Model file for the job. Use its own axes, mm. A direction names the side the tool comes from. Round coordinates to 2 decimals unless told otherwise and drop trailing zeros. Order: outer loops, then holes, each group sorted by start corner. A loop starts at its lowest first (then second) coordinate and runs counter-clockwise, first axis right, second up. Notation, with made-up numbers: M -32.5,8.5 L -7.5,8.5 A14 ccw -7.5,17.5 Z; hole C -22,63.25 d5. An arc over 180 degrees is marked long. Return JSON: item names as keys, results as strings. Group by question number.
Item 1: Slice it at B-B on x = -3.25. Write the cut outline in (y, z).
Item 2: Slice it at C-C on z = 4.25. Write the cut outline in (x, y), then the cut area to 3 significant figures.
Item 3: Slice it at D-D on x = 4.5. Write the cut outline in (y, z), then the cut area to 3 significant figures.
Item 4: Probe line 1 along Y through (x, z) = (5.75, 0.9); line 2 along X through (y, z) = (1.75, 4.7); line 3 along Y through (x, z) = (-3.5, 1.35). List the from-to ranges inside material, lowest first.
Item 5: Pin check, flat tips, straight feed: pin 1 Ø1.2 at (y, z) = (3, 1.5) entering from -X; pin 2 Ø1.7 at (x, y) = (-1, 2) entering from -Z; pin 3 Ø1 at (x, z) = (0, 2) entering from -Y (3 decimals). Stop position of each tip, or through.
Item 6: Slice it at A-A on y = 2.5. Write the cut outline in (x, z), then the cut area to 3 significant figures.
Item 7: Which spindle directions (+Z, -Z, +X, -X, +Y, -Y) get a long thin tool onto all of the face, cutting with end or side? Do faces 1 (the face through (-0.25, 1.75, 5)), 2 (the face through (-2.7, 0.2, 2.3)), 3 (the face through (-3, 0.4, 4)), 4 (the face through (4, 6, 2)). Say none if no direction does.
from build123d import *

# Parameters (mm, degrees)
SM_BASE_FLANGE_1_DEPTH = 6
SKETCH_5_R             = 1
CUT_EXTRUDE_1_DEPTH    = 12.223190277
CUT_EXTRUDE_3_REACH    = 17.683
CUT_EXTRUDE_4_REACH    = 13.223


# Sheet-metal steps are written as plain solids
with BuildPart() as part:
    # Sketch 1 → 基体-法兰1 (new body)
    with BuildSketch(Plane.XY):
        with BuildLine():
            Line((-7, 0), (-1.1366, 0))
            ThreePointArc((-1.1366, 0), (-0.332902433, 0.332902433), (0, 1.1366))
            Line((0, 1.1366), (0, 5.2634))
            ThreePointArc((0, 5.2634), (0.215745145, 5.784254855), (0.7366, 6))
            Line((0.7366, 6), (6, 6))
            Line((6, 6), (6, 6.4))
            Line((6, 6.4), (0.7366, 6.4))
            ThreePointArc((0.7366, 6.4), (-0.067097567, 6.067097567), (-0.4, 5.2634))
            Line((-0.4, 5.2634), (-0.4, 1.1366))
            ThreePointArc((-0.4, 1.1366), (-0.615745145, 0.615745145), (-1.1366, 0.4))
            Line((-1.1366, 0.4), (-7, 0.4))
            Line((-7, 0.4), (-7, 0))
        make_face()
    extrude(amount=SM_BASE_FLANGE_1_DEPTH)

    # 草图5 → 切除-拉伸1 (cut, through all)
    with BuildSketch(Plane(origin=(0, 6.4, 0), x_dir=(1, 0, 0), z_dir=(0, 1, 0))):
        with Locations(Location((2.913465792, -3, 0), (0, 0, 270))):
            Circle(SKETCH_5_R)
    extrude(amount=-CUT_EXTRUDE_1_DEPTH, mode=Mode.SUBTRACT)

    # 草图6 → 切除-拉伸3 (cut, up to next)
    with BuildSketch(Plane.ZY.offset(7), mode=Mode.PRIVATE) as cut_extrude_3_sk1:
        with BuildLine():
            Line((2.3, -3.316111615), (2.3, 3.5366))
            ThreePointArc((2.3, 3.5366), (2.475735931, 3.960864069), (2.9, 4.1366))
            Line((2.9, 4.1366), (3, 4.1366))
            Line((3, 4.1366), (3.1, 4.1366))
            ThreePointArc((3.1, 4.1366), (3.524264069, 3.960864069), (3.7, 3.5366))
            Line((3.7, 3.5366), (3.7, -3.316111615))
            Line((3.7, -3.316111615), (2.3, -3.316111615))
        make_face()
    cut_extrude_3_tool1 = extrude(cut_extrude_3_sk1.sketch, amount=-CUT_EXTRUDE_3_REACH, mode=Mode.PRIVATE) & part.part
    # 草图6 → 切除-拉伸3 (cut, up to next)
    with BuildSketch(Plane.ZY.offset(7), mode=Mode.PRIVATE) as cut_extrude_3_sk2:
        Polygon((1, -3.316111615), (1, 4.1366), (0, 4.629449722), (0, -3.316111615), align=None)
    cut_extrude_3_tool2 = extrude(cut_extrude_3_sk2.sketch, amount=-CUT_EXTRUDE_3_REACH, mode=Mode.PRIVATE) & part.part
    # 草图6 → 切除-拉伸3 (cut, up to next)
    with BuildSketch(Plane.ZY.offset(7), mode=Mode.PRIVATE) as cut_extrude_3_sk3:
        Polygon((5, 4.1366), (6, 4.629449722), (6, -3.316111615), (5, -3.316111615), align=None)
    cut_extrude_3_tool3 = extrude(cut_extrude_3_sk3.sketch, amount=-CUT_EXTRUDE_3_REACH, mode=Mode.PRIVATE) & part.part
    add(cut_extrude_3_tool1.solids().sort_by_distance((-7, 0.356246, 3))[0], mode=Mode.SUBTRACT)
    add(cut_extrude_3_tool2.solids().sort_by_distance((-7, 0.534771, 0.494666))[0], mode=Mode.SUBTRACT)
    add(cut_extrude_3_tool3.solids().sort_by_distance((-7, 0.534771, 5.505334))[0], mode=Mode.SUBTRACT)

    # 草图7 → 切除-拉伸4 (cut, up to next)
    with BuildSketch(Plane.XZ, mode=Mode.PRIVATE) as cut_extrude_4_sk1:
        Polygon((-7, 3.881631359), (-4.559628285, 5), (-7, 5), align=None)
    cut_extrude_4_tool1 = extrude(cut_extrude_4_sk1.sketch, amount=-CUT_EXTRUDE_4_REACH, mode=Mode.PRIVATE) & part.part
    # 草图7 → 切除-拉伸4 (cut, up to next)
    with BuildSketch(Plane.XZ, mode=Mode.PRIVATE) as cut_extrude_4_sk2:
        Polygon((-1.502616723, 5), (-4, 5), (-4.559628285, 5), (-4, 4.7), (-1.502616723, 4.7), align=None)
    cut_extrude_4_tool2 = extrude(cut_extrude_4_sk2.sketch, amount=-CUT_EXTRUDE_4_REACH, mode=Mode.PRIVATE) & part.part
    # 草图7 → 切除-拉伸4 (cut, up to next)
    with BuildSketch(Plane.XZ, mode=Mode.PRIVATE) as cut_extrude_4_sk3:
        Polygon((-7, 2.118368641), (-7, 1), (-4.559628285, 1), align=None)
    cut_extrude_4_tool3 = extrude(cut_extrude_4_sk3.sketch, amount=-CUT_EXTRUDE_4_REACH, mode=Mode.PRIVATE) & part.part
    # 草图7 → 切除-拉伸4 (cut, up to next)
    with BuildSketch(Plane.XZ, mode=Mode.PRIVATE) as cut_extrude_4_sk4:
        Polygon((-4, 1.3), (-4.559628285, 1), (-4, 1), (-1.502616723, 1), (-1.502616723, 1.3), align=None)
    cut_extrude_4_tool4 = extrude(cut_extrude_4_sk4.sketch, amount=-CUT_EXTRUDE_4_REACH, mode=Mode.PRIVATE) & part.part
    add(cut_extrude_4_tool1.solids().sort_by_distance((-6.186543, 0, 4.62721))[0], mode=Mode.SUBTRACT)
    add(cut_extrude_4_tool2.solids().sort_by_distance((-2.895914, 0, 4.855038))[0], mode=Mode.SUBTRACT)
    add(cut_extrude_4_tool3.solids().sort_by_distance((-6.186543, 0, 1.37279))[0], mode=Mode.SUBTRACT)
    add(cut_extrude_4_tool4.solids().sort_by_distance((-2.895914, 0, 1.144962))[0], mode=Mode.SUBTRACT)


solid = part.part
Output values:
{
 "1": {"outline": "M 0,1.3 L 0.4,1.3 L 0.4,2.3 L 0,2.3 Z; M 0,3.7 L 0.4,3.7 L 0.4,4.7 L 0,4.7 Z"},
 "2": {"outline": "M -6.2,0 L -1.14,0 A1.14 ccw 0,1.14 L 0,5.26 A0.74 cw 0.74,6 L 6,6 L 6,6.4 L 0.74,6.4 A1.14 ccw -0.4,5.26 L -0.4,1.14 A0.74 cw -1.14,0.4 L -6.2,0.4 Z", "area": "6.96 mm²"},
 "3": {"outline": "M 6,0 L 6.4,0 L 6.4,6 L 6,6 Z", "area": "2.40 mm²"},
 "4": {"line 1": "6 to 6.4", "line 2": "-0.4 to 0", "line 3": "0 to 0.4"},
 "5": {"pin 1": "x = -0.4", "pin 2": "z = 1", "pin 3": "y = 0.195"},
 "6": {"outline": "M -0.4,1 L 0,1 L 0,2.3 L -0.4,2.3 Z; M -0.4,3.7 L 0,3.7 L 0,5 L -0.4,5 Z", "area": "1.04 mm²"},
 "7": {"face 1": "+Z, +X, -X, -Y", "face 2": "+X, -X, -Y", "face 3": "+Z, -Z, -X, +Y", "face 4": "+Z, -Z, +X, -Y"}
}
